Source: CAD feature listing. Evaluate the final solid. Frame: model axes, mm. Give positions to 0.01 mm unless a question says otherwise; leave off trailing zeros. Order: outer loops, then holes, each group sorted by start corner. A loop starts at its lowest first (then second) coordinate and runs counter-clockwise, first axis right, second up. Notation, with made-up numbers: M 9.5,-10 L 49.5,-10 A17 cw 49.5,17 Z; hole C -13,58 d1. An arc over 180 degrees is marked long. Answer in a Markdown table with one row per item. Add a question column.
(1) Section query B-B, the plane y = -93. Return loops of the section in (x, z) (3 decimals), plus the area to 3 significant figures.
(2) Section query C-C, the plane z = 2.5. Count the separate pieces of the cut face and the enclosed holes in it, plus the area to 3 significant figures.
(3) Pin query (flat end, axial travel): P1, Ø17, axis at x = 472.28, y = 54.77, coming from the +Z side; P2, Ø4, axis at x = -476, z = -2, coming from the -Y side; P3, Ø4, axis at y = 90.5, z = 0, coming from the -X side (3 decimals); P4, Ø4, axis at y = -125.5, z = -0.5, coming from the +X side. Return the tip coordinate at first contact, or that it passes through.
(4) Section query A-A, the plane x = 12. Return loops of the section in (y, z), plus the area to 3 significant figures.
(5) Material intervals for line 1 along X through (y, z) = (-55.5, -1.75) (3 decimals); line 2 along X through (y, z) = (-27, -2.75); line 3 along X through (y, z) = (5, 2.5) (3 decimals), sorted ascending.
from build123d import *

# Parameters (mm, degrees)
BOSS_EXTRUDE1_DEPTH  = 6.35
TABS_DEPTH           = 6.35
FILLET1_R            = 3.175
SKETCH3_R            = 5.3578125
CABLE_TIE_HOLE_DEPTH = 7.35


with BuildPart() as part:
    # Sketch1 → Boss-Extrude1 (new body, symmetric)
    with BuildSketch(Plane.XY):
        with BuildLine():
            Line((-457.2, -109.5375), (457.2, -109.5375))
            ThreePointArc((457.2, -109.5375), (459.44506403, -108.60756403), (460.375, -106.3625))
            Line((460.375, -106.3625), (460.375, 106.3625))
            ThreePointArc((460.375, 106.3625), (459.44506403, 108.60756403), (457.2, 109.5375))
            Line((457.2, 109.5375), (-457.2, 109.5375))
            ThreePointArc((-457.2, 109.5375), (-459.44506403, 108.60756403), (-460.375, 106.3625))
            Line((-460.375, 106.3625), (-460.375, -106.3625))
            ThreePointArc((-460.375, -106.3625), (-459.44506403, -108.60756403), (-457.2, -109.5375))
        make_face()
    extrude(amount=BOSS_EXTRUDE1_DEPTH, both=True)

    # Sketch2 → Tabs (add, symmetric)
    with BuildSketch(Plane.XY):
        with BuildLine():
            Line((-460.375, 80.16875), (-482.6, 80.16875))
            ThreePointArc((-482.6, 80.16875), (-484.84506403, 79.23881403), (-485.775, 76.99375))
            Line((-485.775, 76.99375), (-485.775, 32.54375))
            ThreePointArc((-485.775, 32.54375), (-484.84506403, 30.29868597), (-482.6, 29.36875))
            Line((-482.6, 29.36875), (-460.375, 29.36875))
            Line((-460.375, 29.36875), (-460.375, 80.16875))
        make_face()
        with BuildLine():
            Line((-460.375, -29.36875), (-482.6, -29.36875))
            ThreePointArc((-482.6, -29.36875), (-484.84506403, -30.29868597), (-485.775, -32.54375))
            Line((-485.775, -32.54375), (-485.775, -76.99375))
            ThreePointArc((-485.775, -76.99375), (-484.84506403, -79.23881403), (-482.6, -80.16875))
            Line((-482.6, -80.16875), (-460.375, -80.16875))
            Line((-460.375, -80.16875), (-460.375, -29.36875))
        make_face()
        with BuildLine():
            Line((-370.68125, -109.5375), (-370.68125, -131.7625))
            ThreePointArc((-370.68125, -131.7625), (-369.75131403, -134.00756403), (-367.50625, -134.9375))
            Line((-367.50625, -134.9375), (-323.05625, -134.9375))
            ThreePointArc((-323.05625, -134.9375), (-320.81118597, -134.00756403), (-319.88125, -131.7625))
            Line((-319.88125, -131.7625), (-319.88125, -109.5375))
            Line((-319.88125, -109.5375), (-370.68125, -109.5375))
        make_face()
        with BuildLine():
            Line((-140.49375, -109.5375), (-140.49375, -131.7625))
            ThreePointArc((-140.49375, -131.7625), (-139.56381403, -134.00756403), (-137.31875, -134.9375))
            Line((-137.31875, -134.9375), (-92.86875, -134.9375))
            ThreePointArc((-92.86875, -134.9375), (-90.62368597, -134.00756403), (-89.69375, -131.7625))
            Line((-89.69375, -131.7625), (-89.69375, -109.5375))
            Line((-89.69375, -109.5375), (-140.49375, -109.5375))
        make_face()
    tabs = extrude(amount=TABS_DEPTH, both=True)

    # Mirror1: Tabs across plane
    add(tabs.mirror(Plane(origin=(0, 0, 0), x_dir=(0, 0, 1), z_dir=(1, 0, 0))))

    # Fillet1
    fillet1_edges = [part.edges().sort_by_distance(p)[0] for p in [
        (460.375, -29.36875, 0),
        (460.375, -80.16875, 0),
        (370.68125, -109.5375, 0),
        (319.88125, -109.5375, 0),
        (140.49375, -109.5375, 0),
        (89.69375, -109.5375, 0),
        (-460.375, 29.36875, 0),
        (-460.375, 80.16875, 0),
        (-460.375, -80.16875, 0),
        (-460.375, -29.36875, 0),
        (-319.88125, -109.5375, 0),
        (-370.68125, -109.5375, 0),
        (-89.69375, -109.5375, 0),
        (-140.49375, -109.5375, 0),
        (460.375, 80.16875, 0),
        (460.375, 29.36875, 0),
    ]]
    fillet(fillet1_edges, radius=FILLET1_R)

    # Sketch3 → Cable Tie hole (cut, symmetric)
    with BuildSketch(Plane.XY):
        with Locations((-472.28125, 54.76875)):
            Circle(SKETCH3_R)
        with Locations((-472.28125, -54.76875)):
            Circle(SKETCH3_R)
        with Locations((-345.28125, -121.44375)):
            Circle(SKETCH3_R)
        with Locations((-115.09375, -121.44375)):
            Circle(SKETCH3_R)
    cable_tie_hole = extrude(amount=CABLE_TIE_HOLE_DEPTH, both=True, mode=Mode.SUBTRACT)

    # Mirror2: Cable Tie hole across plane
    add(cable_tie_hole.mirror(Plane(origin=(0, 0, 0), x_dir=(0, 0, 1), z_dir=(1, 0, 0))), mode=Mode.SUBTRACT)


solid = part.part
Values follow:
| question | item | result |
|---|---|---|
| 1 | outline | M -460.375,-6.35 L 460.375,-6.35 L 460.375,6.35 L -460.375,6.35 Z |
| 1 | area | 11,700 mm² |
| 2 | separate pieces | 1 |
| 2 | enclosed holes | 8 |
| 2 | area | 211,000 mm² |
| 3 | P1 | stops at z = 6.35 |
| 3 | P2 | stops at y = -80.17 |
| 3 | P3 | stops at x = -460.375 |
| 3 | P4 | stops at x = 370.68 |
| 4 | outline | M -109.54,-6.35 L 109.54,-6.35 L 109.54,6.35 L -109.54,6.35 Z |
| 4 | area | 2,780 mm² |
| 5 | line 1 | x = -485.775 to -477.589, -466.974 to 466.974, 477.589 to 485.775 |
| 5 | line 2 | x = -460.48 to 460.48 |
| 5 | line 3 | x = -460.375 to 460.375 |
